Source: CAD feature listing. Evaluate the final solid. Frame: model axes, mm. Face numbers are marked on the shaded views. A direction names the side the tool comes from. Give positions to 0.01 mm unless a question says otherwise; leave off trailing zeros. Write each loop counter-clockwise with the first axis right and the second up, starting at its lowest first coordinate (ties: lowest second). Pieces come first, ordered by that corner, then holes. Notation, with made-up numbers: (86, 8) -> (115, 8) arc R23 ccw to (115, 41) -> close; hole circle Ø3 at (7.5, -28.75). An arc over 180 degrees is marked (long way). Write item = value, one per line.
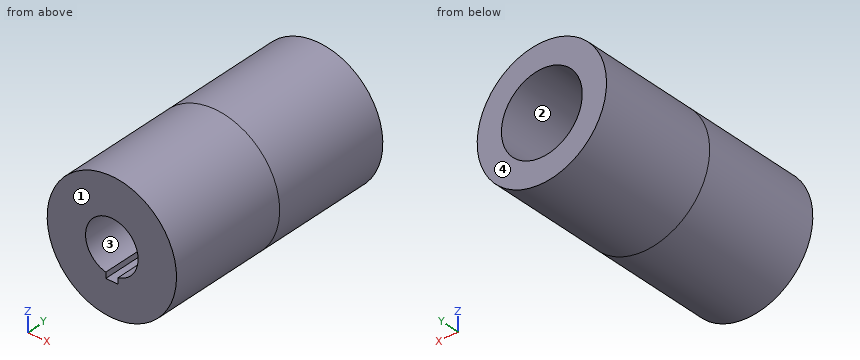
from build123d import *

# Parameters (mm, degrees)
SKETCH1_R           = 16
SKETCH1_R_2         = 10
BOSS_EXTRUDE1_DEPTH = 30
BOSS_EXTRUDE2_START = 30
SKETCH2_R           = 16
BOSS_EXTRUDE2_DEPTH = 30
SKETCH3_R           = 6.5
CUT_EXTRUDE1_DEPTH  = 30
SKETCH4_W           = 3
SKETCH4_H           = 2.5
CUT_EXTRUDE2_DEPTH  = 30


with BuildPart() as part:
    # Sketch1 → Boss-Extrude1 (new body)
    with BuildSketch(Plane(origin=(0, 0, 0), x_dir=(1, 0, 0), z_dir=(0, 1, 0))):
        with Locations(Location((0, 0, 0), (0, 0, 270))):
            Circle(SKETCH1_R)
        with Locations(Location((0, 0, 0), (0, 0, 270))):
            Circle(SKETCH1_R_2, mode=Mode.SUBTRACT)
    extrude(amount=BOSS_EXTRUDE1_DEPTH)

    # Sketch2 → Boss-Extrude2 (add)
    with BuildSketch(Plane.XZ.offset(BOSS_EXTRUDE2_START)):
        with Locations(Location((0, 0, 0), (0, 0, 270))):
            Circle(SKETCH2_R)
    extrude(amount=-BOSS_EXTRUDE2_DEPTH)

    # Sketch3 → Cut-Extrude1 (cut)
    with BuildSketch(Plane.XZ.offset(30)):
        with Locations(Location((0, 0, 0), (0, 0, 270))):
            Circle(SKETCH3_R)
    extrude(amount=-CUT_EXTRUDE1_DEPTH, mode=Mode.SUBTRACT)

    # Sketch4 → Cut-Extrude2 (cut)
    with BuildSketch(Plane.XZ.offset(30)):
        with Locations((0, -6.5)):
            Rectangle(SKETCH4_W, SKETCH4_H)
    extrude(amount=-CUT_EXTRUDE2_DEPTH, mode=Mode.SUBTRACT)


solid = part.part
(1) First-contact query: pin 1 (1 mm diameter, centred on y = 5.5, z = 12.5, fed in from -X); pin 2 (10 mm diameter, centred on y = -22, z = -4.5, fed in from -X); pin 3 (1.6 mm diameter, centred on y = -14.5, z = -7, fed in from +X); pin 4 (18 mm diameter, centred on x = 0, z = 0, fed in from +Y). Flat tips, straight axial feed; report the tip coordinate or a pass-through.
Values follow:
pin_1 = -10.58
pin_2 = -16
pin_3 = 14.75
pin_4 = 0
(2) Access query for the marked faces 1 and 2. Directions: +Z, -Z, +X, -X, +Y, -Y. A direction counts if a zero-diameter tool reaches every point of the face in a straight line with its end or side. Return the directions, or none.
Values follow:
face_1 = +Z, -Z, +X, -X, -Y
face_2 = +Y
(3) Material intervals for line 1 (X direction, y = 8, z = 0); line 2 (Z direction, x = 0, y = -6); line 3 (X direction, y = -17, z = 0), sorted ascending.
Values follow:
line_1 = -16 to -10, 10 to 16
line_2 = -16 to -7.75, 6.5 to 16
line_3 = -16 to -6.5, 6.5 to 16
(4) Section query C-C (y = -19.5). Return loops of the section in (x, z).
Values follow:
outline = circle Ø32 at (0, 0); hole (-1.5, -7.75) -> (1.5, -7.75) -> (1.5, -6.32) arc R6.5 ccw (long way) to (-1.5, -6.32) -> close
(5) Pull-direction query (X, two-part tool) for the marked faces 3 and 4; classes: pulls with the +X half, pulls with the -X half, needs draft (parallel to the pull), parting line crosses it, or undercut.
Values follow:
face_3 = undercut
face_4 = needs draft
(6) Section query B-B (z = 0). Return loops of the section in (x, y).
Values follow:
outline = (-16, -30) -> (-6.5, -30) -> (-6.5, 0) -> (-10, 0) -> (-10, 30) -> (-16, 30) -> close; (6.5, -30) -> (16, -30) -> (16, 30) -> (10, 30) -> (10, 0) -> (6.5, 0) -> close
(7) Section query D-D (x = 8). Return loops of the section in (y, z), plus the area to 3 significant figures.
Values follow:
outline = (-30, -13.86) -> (30, -13.86) -> (30, -6) -> (0, -6) -> (0, 6) -> (30, 6) -> (30, 13.86) -> (-30, 13.86) -> close
area = 1,300 mm2
(8) Section query A-A (x = 0). Return loops of the section in (y, z).
Values follow:
outline = (-30, -16) -> (30, -16) -> (30, -10) -> (0, -10) -> (0, -7.75) -> (-30, -7.75) -> close; (-30, 6.5) -> (0, 6.5) -> (0, 10) -> (30, 10) -> (30, 16) -> (-30, 16) -> close
